from build123d import *

# Parameters (mm, degrees)
SKETCH1_W                 = 50
SKETCH1_H                 = 95
BOSS_EXTRUDE1_DEPTH       = 9.525
F_4_0MM_DOWEL_HOLE1_D     = 4
F_4_0MM_DOWEL_HOLE1_DEPTH = 3.2
F_4_0MM_DOWEL_HOLE1_TIP   = 1.201721238
F_4_0MM_DOWEL_HOLE2_D     = 4
F_4_0MM_DOWEL_HOLE2_DEPTH = 3.2
F_4_0MM_DOWEL_HOLE2_TIP   = 1.201721238


with BuildPart() as part:
    # Sketch1 → Boss-Extrude1 (new body)
    with BuildSketch(Plane.XY):
        Rectangle(SKETCH1_W, SKETCH1_H)
    extrude(amount=-BOSS_EXTRUDE1_DEPTH)

    # Ø4.0mm Dowel Hole1
    with Locations(Plane(origin=(0, 47.5, 0), x_dir=(1, 0, 0), z_dir=(0, 1, 0))):
        with Locations((0, 4.7625), (16.67, 4.7625), (-16.67, 4.7625)):
            Hole(F_4_0MM_DOWEL_HOLE1_D / 2, depth=F_4_0MM_DOWEL_HOLE1_DEPTH)
            with Locations((0, 0, -(F_4_0MM_DOWEL_HOLE1_DEPTH + F_4_0MM_DOWEL_HOLE1_TIP / 2))):  # 118° drill point
                Cone(0, F_4_0MM_DOWEL_HOLE1_D / 2, F_4_0MM_DOWEL_HOLE1_TIP, mode=Mode.SUBTRACT)

    # Ø4.0mm Dowel Hole2
    with Locations(Plane.XZ.offset(47.5)):
        with Locations((16.67, -4.7625), (0, -4.7625), (-16.67, -4.7625)):
            Hole(F_4_0MM_DOWEL_HOLE2_D / 2, depth=F_4_0MM_DOWEL_HOLE2_DEPTH)
            with Locations((0, 0, -(F_4_0MM_DOWEL_HOLE2_DEPTH + F_4_0MM_DOWEL_HOLE2_TIP / 2))):  # 118° drill point
                Cone(0, F_4_0MM_DOWEL_HOLE2_D / 2, F_4_0MM_DOWEL_HOLE2_TIP, mode=Mode.SUBTRACT)


solid = part.part
Geometry: final body of the model. Coordinates: model frame, mm. A direction names the side the tool comes from. Round coordinates to 2 decimals unless told otherwise and drop trailing zeros. Put each result on its own line as item: value. Start each with the question number.
(1) Contact query for flat-ended pins moving along their axis: pin 1 Ø3 at (x, z) = (-16.67, -4.76) entering from +Y; pin 2 Ø3.5 at (x, z) = (16.67, -4.76) entering from +Y; pin 3 Ø2.5 at (x, z) = (0, -4.76) entering from -Y. Output: stop coordinate, or through.
(2) Draft query along Z for faces 1 (the face through (0, 1, 0)), 2 (the face through (-18.58, 45.88, -5.36)), 3 (the face through (-25, -1, -5)). Return one class per face: +Z half, -Z half, draft (parallel to the pull), parting line (faces both ways), or undercut.
(3) Material intervals for line 1 along Z through (x, y) = (0, 45.35) (1 decimal); line 2 along Z through (x, y) = (0, -44) (3 decimals); line 3 along Y through (x, z) = (-17, -3.75), sorted ascending. Write a range as [from, to].
(4) Set-up query: faces 4 (the face through (-1.91, 45.88, -5.36)), 5 (the face through (-18.578, -45.878, -4.162)), 6 (the face through (0, -47.5, -7)). Return all of +Z, -Z, +X, -X, +Y, -Y with unobstructed straight access to the full face (end or side cutting, diameter ignored); none if empty.
Findings below:
1. pin 1: stops at y = 44
1. pin 2: stops at y = 44.15
1. pin 3: stops at y = -43.85
2. face 1: +Z half
2. face 2: undercut
2. face 3: draft
3. line 1: z = [-9.5, -6.8], [-2.8, 0]
3. line 2: z = [-9.525, -6.263], [-3.262, 0]
3. line 3: y = [-43.74, 43.74]
4. face 4: +Y
4. face 5: -Y
4. face 6: +Z, -Z, +X, -X, -Y
